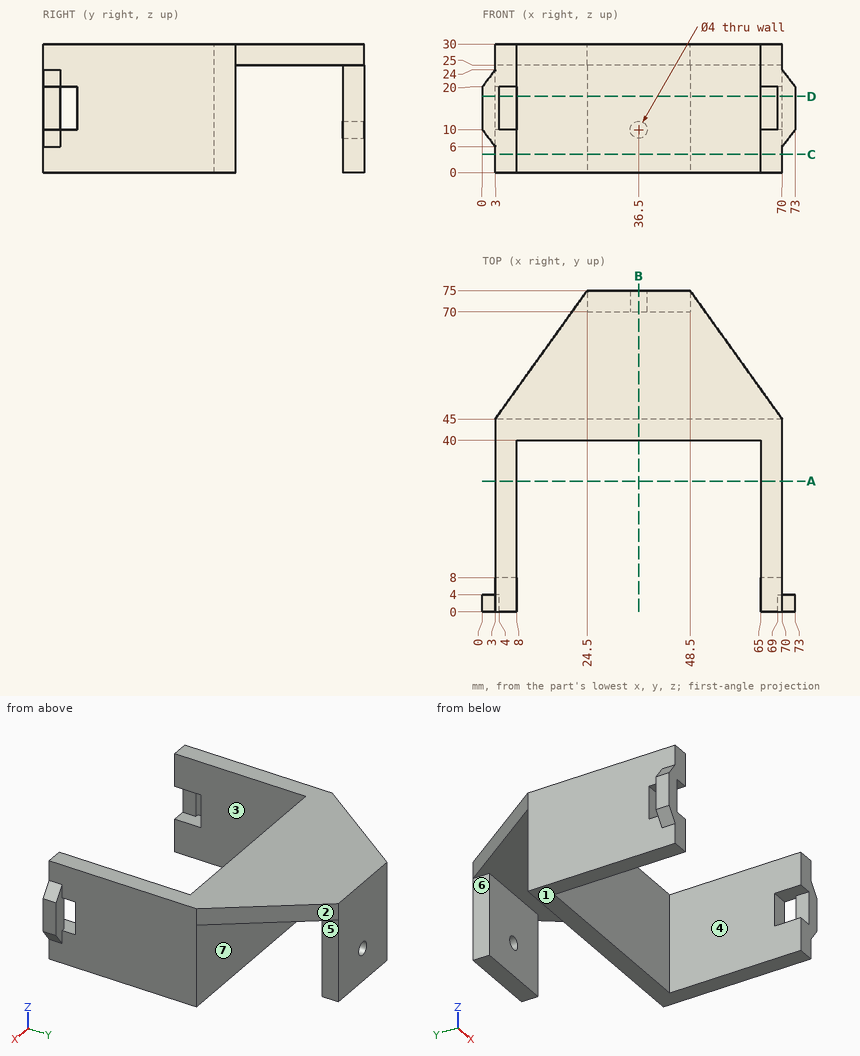
Here's the drawing with two shaded views (mm, measured from the low corner). I have some questions. A direction names the side the tool comes from. Coordinates: 2 decimals unless noted, no trailing zeros. Order: outer loops, then holes, each group sorted by start corner. A loop starts at its lowest first (then second) coordinate and runs counter-clockwise, first axis right, second up. Notation, with made-up numbers: M 49,2.5 L 62,2.5 A11 cw 62,10.5 Z; hole C -16.5,22.5 d5. An arc over 180 degrees is marked long. Write item = value, one per line.
(1) I need wall thicknesses on line 1 along X through (y, z) = (17, 9); line 2 along Y through (x, z) = (27.5, 14.5); line 3 along Z through (x, y) = (36.5, 71.6). Which ranges of each line are inside material? Lowest first, please. Write a range as [from, to].
Results are:
line_1 = [3, 8], [65, 70]
line_2 = [40, 45], [70, 75]
line_3 = [0, 8], [12, 30]
(2) For pin 1 Ø2.5 at (x, z) = (67, 13.5) entering from -Y; pin 2 Ø5 at (x, z) = (36.5, 10) entering from -Y; pin 3 Ø2 at (y, z) = (1.5, 15.5) entering from -X; pin 4 Ø5.5 at (y, z) = (73.5, 17) entering from +X, each with a flat end and sliding along its axis, tell me the tip position at first contact or that it passes through.
Results are:
pin_1 = 8
pin_2 = 40
pin_3 = 0
pin_4 = 48.5
(3) Suppose I cut it at C-C on z = 4.25. Please give me the cut outline in (x, y), plus the area to 3 significant figures.
Results are:
outline = M 3,0 L 8,0 L 8,40 L 65,40 L 65,0 L 70,0 L 70,45 L 3,45 Z; M 24.5,70 L 48.5,70 L 48.5,75 L 24.5,75 Z
area = 855 mm2
(4) Suppose I cut it at B-B on x = 36.5. Please give me the cut outline in (y, z), plus the area to 3 significant figures.
Results are:
outline = M 40,0 L 45,0 L 45,25 L 70,25 L 70,12 L 75,12 L 75,30 L 40,30 Z; M 70,0 L 75,0 L 75,8 L 70,8 Z
area = 405 mm2
(5) Suppose I cut it at D-D on z = 17.75. Please give me the cut outline in (x, y).
Results are:
outline = M 0,0 L 4,0 L 4,4 L 0,4 Z; M 3,8 L 8,8 L 8,40 L 65,40 L 65,8 L 70,8 L 70,45 L 3,45 Z; M 24.5,70 L 48.5,70 L 48.5,75 L 24.5,75 Z; M 69,0 L 73,0 L 73,4 L 69,4 Z
(6) Suppose I cut it at A-A on y = 30.5. Please give me the cut outline in (x, z), plus the area to 3 significant figures.
Results are:
outline = M 3,0 L 8,0 L 8,30 L 3,30 Z; M 65,0 L 70,0 L 70,30 L 65,30 Z
area = 300 mm2
(7) If we mould it in two halves opening along X, with no side actions, what happens to the marked faces 1, 2 and 3? For each: pulls with the +X half, pulls with the -X half, needs draft (parallel to the pull), parting line crosses it, or undercut.
Results are:
face_1 = needs draft
face_2 = pulls with the +X half
face_3 = undercut
(8) For the marked faces 4, 5, 6 and 7, which set-ups out of +Z, -Z, +X, -X, +Y, -Y let a thin tool reach every point of the face, with its end or its side?
Results are:
face_4 = +Z, -Z, -Y
face_5 = -Z, +X, +Y
face_6 = -Z, -X, +Y
face_7 = -Z, +X, -X
